from build123d import *

# Parameters (mm, degrees)
SKETCH_W     = 18
SKETCH_H     = 33.5
PAD_DEPTH    = 1.6
FILLET_R     = 1
SKETCH001_W  = 9.16
SKETCH001_H  = 6.5
POCKET_DEPTH = 5


with BuildPart() as part:
    # Sketch → Pad (new body)
    with BuildSketch(Plane.XY):
        Rectangle(SKETCH_W, SKETCH_H)
    extrude(amount=PAD_DEPTH)

    # Fillet
    fillet_edges = [part.edges().sort_by_distance(p)[0] for p in [
        (9, 16.75, 0.8),
        (9, -16.75, 0.8),
        (-9, -16.75, 0.8),
        (-9, 16.75, 0.8),
    ]]
    fillet(fillet_edges, radius=FILLET_R)

    # Sketch001 → Pocket (cut)
    with BuildSketch(Plane.XY):
        with Locations((0, 14.45)):
            Rectangle(SKETCH001_W, SKETCH001_H)
    extrude(amount=POCKET_DEPTH, mode=Mode.SUBTRACT)


solid = part.part
The model under review builds one solid part; all positions refer to its coordinate system, in mm. A direction names the side the tool comes from. Round coordinates to 2 decimals unless told otherwise and drop trailing zeros. Order: outer loops, then holes, each group sorted by start corner. A loop starts at its lowest first (then second) coordinate and runs counter-clockwise, first axis right, second up. Notation, with made-up numbers: (38, -15) -> (57, -15) arc R26 cw to (57, 10) -> close; hole circle Ø9 at (28.5, 73.5). An arc over 180 degrees is marked (long way). Write item = value, one per line. Start each with the question number.
Item 1: Clearance check with a flat-ended pin moving along its axis: pin 1 Ø0.5 at (x, z) = (0.5, 0.5) entering from +Y. State where the tip first meets the part, or that it passes through.
Item 2: Consider section A-A on z = 0.75. Write out the cut boundary in (x, y), plus the area to 3 significant figures.
Item 3: Consider section B-B on x = -3.5. Write out the cut boundary in (y, z).
Item 4: For faces 4 (the face through (0, 11.2, 1)), 5 (the face through (9, 0, 1)), list the 3-axis set-ups (+Z, -Z, +X, -X, +Y, -Y) from which the entire face can be reached by the end or side of a thin tool; tool diameter is ignored.
Item 5: Mouldability with a two-part tool opening along X and no side actions: class faces 1 (the face through (0, 0, 1.6)), 2 (the face through (-4.58, 14, 1)), 3 (the face through (8.699, -16.465, 0.811)) as released by +X, released by -X, zero draft, split by the parting line, or undercut.
Item 6: For line 1 along X through (y, z) = (13.5, 1.45); line 2 along Y through (x, z) = (-3.75, 0.5); line 3 along Y through (x, z) = (8.25, 0.8), list the stretches that pass through material, from the lowest coordinate up.
Conclusion:
q1.pin_1 = 11.2
q2.outline = (-9, -15.75) arc R1 ccw to (-8, -16.75) -> (8, -16.75) arc R1 ccw to (9, -15.75) -> (9, 15.75) arc R1 ccw to (8, 16.75) -> (4.58, 16.75) -> (4.58, 11.2) -> (-4.58, 11.2) -> (-4.58, 16.75) -> (-8, 16.75) arc R1 ccw to (-9, 15.75) -> close
q2.area = 551 mm2
q3.outline = (-16.75, 0) -> (11.2, 0) -> (11.2, 1.6) -> (-16.75, 1.6) -> close
q4.face_4 = +Z, -Z, +Y
q4.face_5 = +Z, -Z, +X, +Y, -Y
q5.face_1 = zero draft
q5.face_2 = undercut
q5.face_3 = released by +X
q6.line_1 = -9 to -4.58, 4.58 to 9
q6.line_2 = -16.75 to 11.2
q6.line_3 = -16.72 to 16.72
